Geometry: final body of the model. Coordinates: model frame, mm. Give positions to 0.01 mm unless a question says otherwise; leave off trailing zeros. Write each loop counter-clockwise with the first axis right and the second up, starting at its lowest first coordinate (ties: lowest second). Pieces come first, ordered by that corner, then holes. Notation, with made-up numbers: M 33,28 L 51,28 A19 ccw 51,48 Z; hole C -4,-20.5 d4. An arc over 180 degrees is marked long. Use a Markdown table: item, result. Add a question column.
(1) Material intervals for L1, parallel to Y at x = -1, z = -15; L2, parallel to Z at x = -0.75, y = -173; L3, parallel to Y at x = -5.25, z = -1154, sorted ascending.
(2) Cut plane A-A (z = -530.5). Output: boundary loops of the cut face in (x, y), plus the area to 3 significant figures.
(3) Pin query (flat end, axial travel): pin 1 Ø4 at (y, z) = (-153, -473) entering from -X; pin 2 Ø3.5 at (y, z) = (-173, -120) entering from +X. Return the tip coordinate at first contact, or that it passes through.
(4) Cut plane C-C (y = -44.5). Output: boundary loops of the cut face in (x, z).
(5) Cut plane B-B (x = -5.5). Output: boundary loops of the cut face in (y, z).
(6) Draft query along Y for faces 1 (the flat face through (0, -89, -781)), 2 (the flat face through (-1.5, -92, -781)). Return one class per face: released by +Y, released by -Y, zero draft, split by the parting line, or undercut.
```python
from build123d import *

# Parameters (mm, degrees)
BOSS_EXTRUDE1_DEPTH            = 1585
FILLET1_R                      = 1.5
F_4_5_4_5_DIAMETER_HOLE1_D     = 4.5
F_4_5_4_5_DIAMETER_HOLE1_DEPTH = 1.5
LPATTERN2_COUNT                = 2
LPATTERN2_PITCH                = 166


with BuildPart() as part:
    # Sketch1 → Boss-Extrude1 (new body)
    with BuildSketch(Plane.XY):
        Polygon((-10, -1.5), (-10, 0), (0, 0), (0, -181), (-10, -181), (-10, -179.5), (-1.5, -179.5), (-1.5, -1.5), align=None)
    extrude(amount=-BOSS_EXTRUDE1_DEPTH)

    # Fillet1
    fillet1_edges = [part.edges().sort_by_distance(p)[0] for p in [
        (0, -181, -792.5),
        (0, 0, -792.5),
    ]]
    fillet(fillet1_edges, radius=FILLET1_R)

    # Ø4.5 (4.5) Diameter Hole1
    with Locations(Plane(origin=(0, 0, 0), x_dir=(0, 0, -1), z_dir=(1, 0, 0))):
        with Locations((15, -7), (120, -7), (1555, -7)):
            f_4_5_4_5_diameter_hole1 = Hole(F_4_5_4_5_DIAMETER_HOLE1_D / 2, depth=F_4_5_4_5_DIAMETER_HOLE1_DEPTH)

    # LPattern2: Ø4.5 (4.5) Diameter Hole1 ×2
    with Locations(*[(0, -i * LPATTERN2_PITCH, 0) for i in range(1, LPATTERN2_COUNT)]):
        add(f_4_5_4_5_diameter_hole1, mode=Mode.SUBTRACT)


solid = part.part
```
Answer list:
| question | item | result |
|---|---|---|
| 1 | L1 | -180.91 to -175.25, -170.75 to -9.25, -4.75 to -0.09 |
| 1 | L2 | -1585 to -1557.25, -1552.75 to -122.25, -117.75 to -17.25, -12.75 to 0 |
| 1 | L3 | -181 to -179.5, -1.5 to 0 |
| 2 | outline | M -10,-181 L -1.5,-181 A1.5 ccw 0,-179.5 L 0,-1.5 A1.5 ccw -1.5,0 L -10,0 L -10,-1.5 L -1.5,-1.5 L -1.5,-179.5 L -10,-179.5 Z |
| 2 | area | 296 mm² |
| 3 | pin 1 | x = -1.5 |
| 3 | pin 2 | through |
| 4 | outline | M -1.5,-1585 L 0,-1585 L 0,0 L -1.5,0 Z |
| 5 | outline | M -181,-1585 L -179.5,-1585 L -179.5,0 L -181,0 Z; M -1.5,-1585 L 0,-1585 L 0,0 L -1.5,0 Z |
| 6 | face 1 | zero draft |
| 6 | face 2 | undercut |
